The listing builds one solid part. Answer for the finished solid, in the listing's coordinates (mm). Give positions to 0.01 mm unless a question says otherwise; leave off trailing zeros. Loops run counter-clockwise (first coordinate to the right, second up) from the corner with the lowest first, then second, coordinate; pieces in that order, holes last. Notation, with made-up numbers: M -39,14 L -5,14 A21 cw -5,36 Z; hole C 6.5,-7 d1. An arc over 180 degrees is marked long. Return JSON: item names as keys, results as strings.
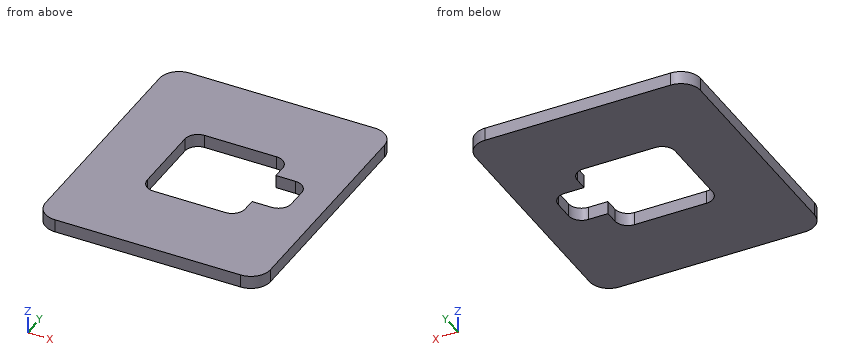
from build123d import *

# Parameters (mm, degrees)
SKETCH_W      = 34.5
SKETCH_H      = 39.5
EXTRUDE_DEPTH = 2
FILLET_R      = 3
FILLET001_R   = 2


with BuildPart() as part:
    # Sketch → Extrude (new body)
    with BuildSketch(Plane.XY):
        Rectangle(SKETCH_W, SKETCH_H)
        Polygon((-7.5, -7.5), (-7.5, 7.5), (7.5, 7.5), (7.5, 3.5), (12.5, 3.5), (12.5, -3.5), (7.5, -3.5), (7.5, -7.5), align=None, mode=Mode.SUBTRACT)
    extrude(amount=EXTRUDE_DEPTH)

    # Fillet
    fillet_edges = [part.edges().sort_by_distance(p)[0] for p in [
        (-17.25, -19.75, 1),
        (-17.25, 19.75, 1),
        (17.25, 19.75, 1),
        (17.25, -19.75, 1),
    ]]
    fillet(fillet_edges, radius=FILLET_R)

    # Fillet001
    fillet001_edges = [part.edges().sort_by_distance(p)[0] for p in [
        (-7.5, -7.5, 1),
        (-7.5, 7.5, 1),
        (7.5, 7.5, 1),
        (12.5, 3.5, 1),
        (12.5, -3.5, 1),
        (7.5, -7.5, 1),
    ]]
    fillet(fillet001_edges, radius=FILLET001_R)


solid = part.part
(1) The part is cut by section C-C (y = -5). Determine the outline of the cut face in (x, z).
Values follow:
{"outline": "M -17.25,0 L -7.5,0 L -7.5,2 L -17.25,2 Z; M 7.5,0 L 17.25,0 L 17.25,2 L 7.5,2 Z"}
(2) The part is cut by section A-A (x = 2). Determine the outline of the cut face in (y, z), and give its area (3 significant figures).
Values follow:
{"outline": "M -19.75,0 L -7.5,0 L -7.5,2 L -19.75,2 Z; M 7.5,0 L 19.75,0 L 19.75,2 L 7.5,2 Z", "area": "49.0 mm²"}
(3) Straight lines are drawn through the part: line 1 along X through (y, z) = (-0.5, 0.35); line 2 along Y through (x, z) = (8, 1.8); line 3 along Y through (x, z) = (-2.5, 1.85). For each, find the intervals that lie inside material, in ascending order.
Values follow:
{"line 1": "-17.25 to -7.5, 12.5 to 17.25", "line 2": "-19.75 to -3.5, 3.5 to 19.75", "line 3": "-19.75 to -7.5, 7.5 to 19.75"}
(4) The part is cut by section B-B (z = 0.45). Determine the outline of the cut face in (x, y).
Values follow:
{"outline": "M -17.25,-16.75 A3 ccw -14.25,-19.75 L 14.25,-19.75 A3 ccw 17.25,-16.75 L 17.25,16.75 A3 ccw 14.25,19.75 L -14.25,19.75 A3 ccw -17.25,16.75 Z; hole M -7.5,-5.5 A2 ccw -5.5,-7.5 L 5.5,-7.5 A2 ccw 7.5,-5.5 L 7.5,-3.5 L 10.5,-3.5 A2 ccw 12.5,-1.5 L 12.5,1.5 A2 ccw 10.5,3.5 L 7.5,3.5 L 7.5,5.5 A2 ccw 5.5,7.5 L -5.5,7.5 A2 ccw -7.5,5.5 Z"}
